Print and shaded views of the part. All mm, measured from the part's lowest x, y and z. A direction names the side the tool comes from. Coordinates: 2 decimals unless noted, no trailing zeros. Order: outer loops, then holes, each group sorted by start corner. A loop starts at its lowest first (then second) coordinate and runs counter-clockwise, first axis right, second up. Notation, with made-up numbers: M 74,17.5 L 112,17.5 A22 cw 112,52.5 Z; hole C 2,10.5 d11. An arc over 180 degrees is marked long. Return JSON: item names as keys, results as strings.
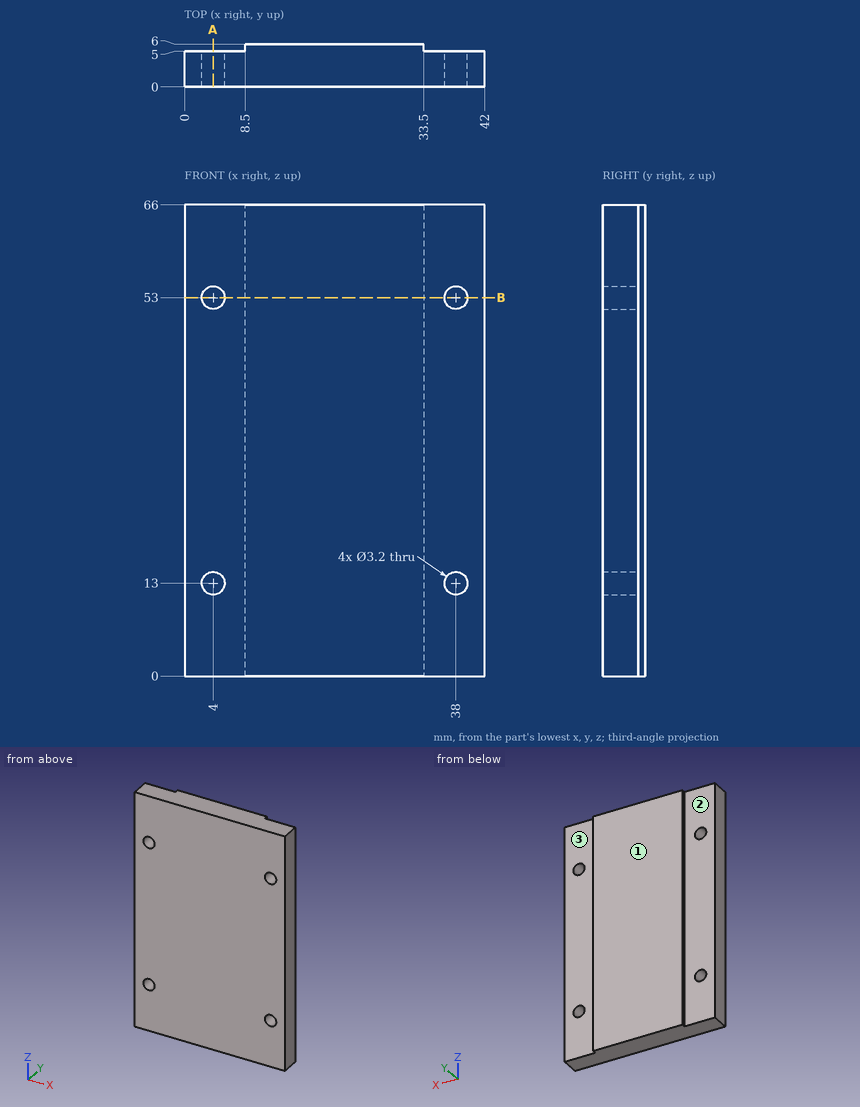
Item 1: Saw through at A-A (x = 4). Write the cut outline in (y, z), and give its area (3 significant figures).
Check result:
{"outline": "M 0,0 L 5,0 L 5,11.4 L 0,11.4 Z; M 0,14.6 L 5,14.6 L 5,51.4 L 0,51.4 Z; M 0,54.6 L 5,54.6 L 5,66 L 0,66 Z", "area": "298 mm2"}
Item 2: 3-axis set-ups, long thin cutter, end or side, ignore diameter. For the marked faces 1, 2 and 3: which of +Z, -Z, +X, -X, +Y, -Y reach the whole face in a straight line?
Check result:
{"face 1": "+Z, -Z, +X, -X, +Y", "face 2": "+Z, -Z, -X, +Y", "face 3": "+Z, -Z, +X, +Y"}
Item 3: Wall check: line 1 (Z direction, x = 38, y = 3.6); line 2 (X direction, y = 3.35, z = 53); line 3 (X direction, y = 5.6, z = 46.5). Give the ranges that are in metal, low to high.
Check result:
{"line 1": "z = 0 to 11.4, 14.6 to 51.4, 54.6 to 66", "line 2": "x = 0 to 2.4, 5.6 to 36.4, 39.6 to 42", "line 3": "x = 8.5 to 33.5"}
Item 4: Saw through at B-B (z = 53). Write the cut outline in (x, y), and give its area (3 significant figures).
Check result:
{"outline": "M 0,0 L 2.4,0 L 2.4,5 L 0,5 Z; M 5.6,0 L 36.4,0 L 36.4,5 L 33.5,5 L 33.5,6 L 8.5,6 L 8.5,5 L 5.6,5 Z; M 39.6,0 L 42,0 L 42,5 L 39.6,5 Z", "area": "203 mm2"}
Item 5: Drop flat-ended pins along their axis: pin 1 Ø2 at (x, y) = (14.5, 4.5) entering from -Z; pin 2 Ø2.5 at (x, z) = (38, 53) entering from +Y; pin 3 Ø4 at (x, z) = (39, 49) entering from +Y; pin 4 Ø0.5 at (y, z) = (5.5, 18.5) entering from -X. Give the stop position or say it passes through.
Check result:
{"pin 1": "stops at z = 0", "pin 2": "passes through", "pin 3": "stops at y = 5", "pin 4": "stops at x = 8.5"}
